```python
from build123d import *

# Parameters (mm, degrees)
BOSS_EXTRUDE1_DEPTH = 5
SKETCH3_W           = 182
SKETCH3_H           = 142.11
SKETCH3_W_2         = 177
SKETCH3_H_2         = 137.11
BOSS_EXTRUDE2_DEPTH = 10
SKETCH6_R           = 2
CUT_EXTRUDE3_DEPTH  = 211
SKETCH8_R           = 2
CUT_EXTRUDE4_DEPTH  = 211


with BuildPart() as part:
    # Sketch1 → Boss-Extrude1 (new body)
    with BuildSketch(Plane(origin=(0, 0, 0), x_dir=(1, 0, 0), z_dir=(0, 1, 0))):
        Polygon((-95, 75.055), (95, 75.055), (95, 10), (115, 10), (115, -10), (95, -10), (95, -75.055), (-95, -75.055), (-95, -10), (-115, -10), (-115, 10), (-95, 10), align=None)
    extrude(amount=BOSS_EXTRUDE1_DEPTH)

    # Sketch3 → Boss-Extrude2 (add)
    with BuildSketch(Plane(origin=(0, 5, 0), x_dir=(1, 0, 0), z_dir=(0, 1, 0))):
        Rectangle(SKETCH3_W, SKETCH3_H)
        Rectangle(SKETCH3_W_2, SKETCH3_H_2, mode=Mode.SUBTRACT)
    extrude(amount=BOSS_EXTRUDE2_DEPTH)

    # Sketch6 → Cut-Extrude3 (cut)
    with BuildSketch(Plane(origin=(0, 0, -75.055), x_dir=(-1, 0, 0), z_dir=(0, 0, -1))):
        with Locations((65, 10)):
            Circle(SKETCH6_R)
        with Locations((0, 10)):
            Circle(SKETCH6_R)
        with Locations((-65, 10)):
            Circle(SKETCH6_R)
    extrude(amount=-CUT_EXTRUDE3_DEPTH, mode=Mode.SUBTRACT)

    # Sketch8 → Cut-Extrude4 (cut)
    with BuildSketch(Plane.ZY.offset(95)):
        with Locations(Location((55.055, 10, 0), (0, 0, 180))):
            Circle(SKETCH8_R)
        with Locations(Location((0, 10, 0), (0, 0, 180))):
            Circle(SKETCH8_R)
        with Locations(Location((-55.055, 10, 0), (0, 0, 180))):
            Circle(SKETCH8_R)
    extrude(amount=-CUT_EXTRUDE4_DEPTH, mode=Mode.SUBTRACT)


solid = part.part
```
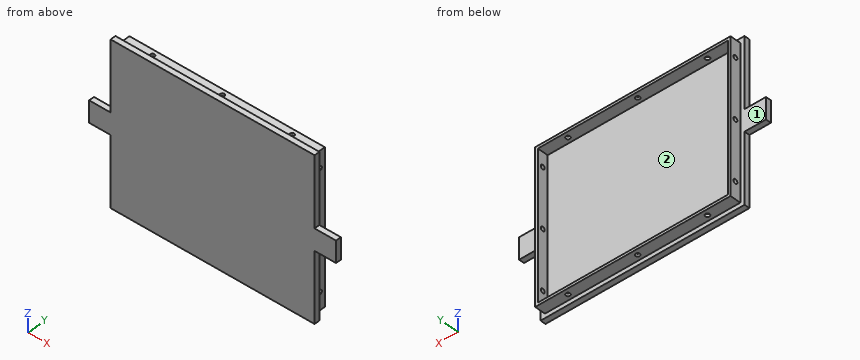
Could you check a few things on this model? Use its own coordinates, in mm. Face numbers are marked on the shaded views. Round coordinates to 2 decimals unless told otherwise and drop trailing zeros. Loops run counter-clockwise (first coordinate to the right, second up) from the corner with the lowest first, then second, coordinate; pieces in that order, holes last. Notation, with made-up numbers: M -12.5,19 L 28.5,19 A9 ccw 28.5,34 Z; hole C -22.75,-6.5 d10. An arc over 180 degrees is marked long. Answer as CSV lines item,"result".
1) If I drill on probe 1 along Z at (x, y) = (-89.55, 10) (3 decimals); probe 2 along X at (y, z) = (14, 54.5); probe 3 along Z at (x, y) = (-54, 8.25) (3 decimals), over which ranges is the centre line in solid material (lowest first)?
From the geometry:
probe 1,"-71.055 to -57.055, -53.055 to -2, 2 to 53.055, 57.055 to 71.055"
probe 2,"-91 to -88.5, 88.5 to 91"
probe 3,"-71.055 to -68.555, 68.555 to 71.055"
2) Imagine slicing it at A-A on x = 58. List the corners of the cut face in (y, z) for me (3 decimals).
From the geometry:
outline,"M 0,-75.055 L 5,-75.055 L 5,-71.055 L 15,-71.055 L 15,-68.555 L 5,-68.555 L 5,68.555 L 15,68.555 L 15,71.055 L 5,71.055 L 5,75.055 L 0,75.055 Z"
3) We'd pull the mould along X, two halves only. Please class the marked faces 1 and 2: released by +X, released by -X, zero draft, split by the parting line, or undercut.
From the geometry:
face 1,"zero draft"
face 2,"undercut"
4) Imagine slicing it at B-B on z = -15. List the corners of the cut face in (x, y) for me.
From the geometry:
outline,"M -95,0 L 95,0 L 95,5 L 91,5 L 91,15 L 88.5,15 L 88.5,5 L -88.5,5 L -88.5,15 L -91,15 L -91,5 L -95,5 Z"
5) For pin 1 Ø1.5 at (y, z) = (6, 30) entering from -X; pin 2 Ø8 at (y, z) = (2, 57) entering from +X; pin 3 Ø4.5 at (x, y) = (-65, 10) entering from -Z (3 decimals), each with a flat end and sliding along its axis, tell me the tip position at first contact or that it passes through.
From the geometry:
pin 1,"x = -91"
pin 2,"x = 95"
pin 3,"z = -71.055"
